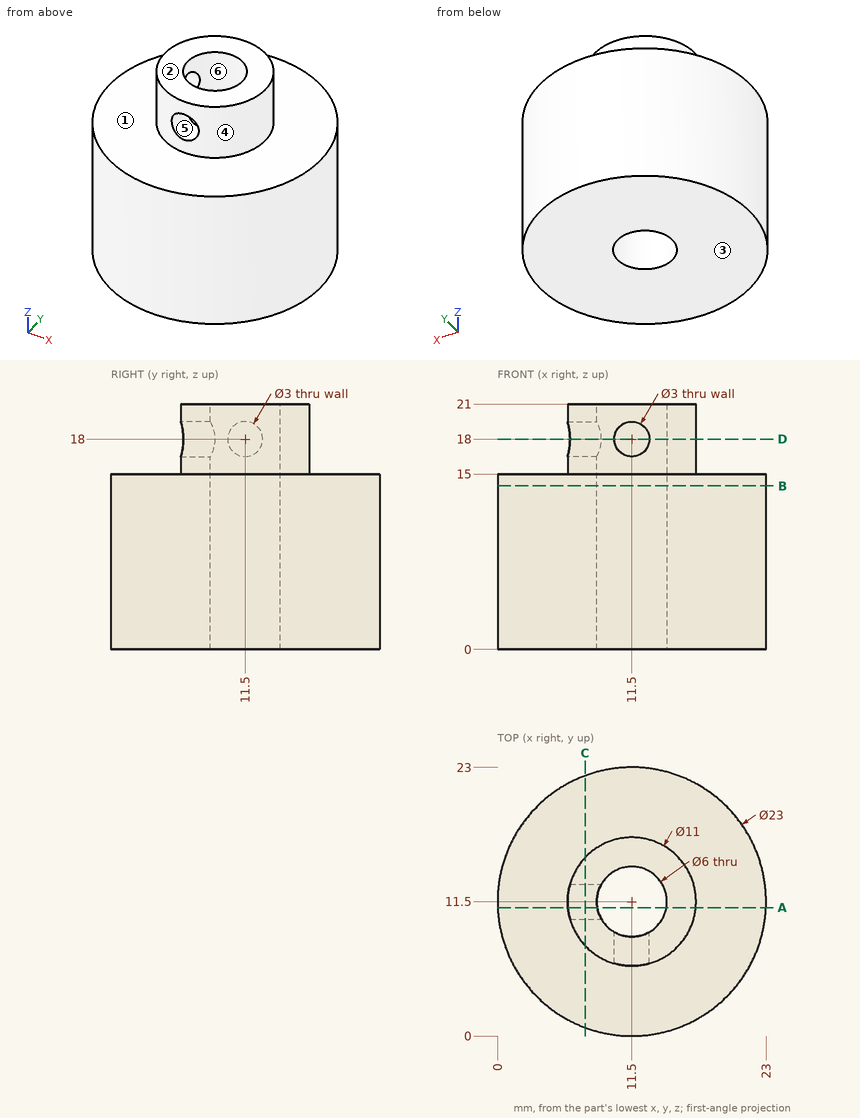
Check sheet for the drawn part. Datum: minimum x, y, z corner. Units: mm. A direction names the side the tool comes from. Round coordinates to 2 decimals unless told otherwise and drop trailing zeros. Order: outer loops, then holes, each group sorted by start corner. A loop starts at its lowest first (then second) coordinate and runs counter-clockwise, first axis right, second up.
(1) Cross-section at A-A, the plane y = 11. Enter the section's corners in (x, z).
(2) Access from +Z, -Z, +X, -X, +Y, -Y to the whole of each face (thin tool, end or side, straight path). Record for the marked faces 1 and 2.
(3) Cross-section at C-C, the plane x = 7.5. Enter the section's corners in (y, z).
(4) Cross-section at B-B, the plane z = 14. Enter the section's corners in (x, y), and give its area (3 significant figures).
(5) Go/stop test with flat-tipped pins: P1, Ø1, axis at x = 16, z = 17.5, coming from the +Y side; P2, Ø4, axis at y = 20.5, z = 10.5, coming from the -X side; P3, Ø10, axis at y = 17.5, z = 15.5, coming from the -X side. Record where each tip stops, or that it passes through.
(6) Draft check along X on the marked faces 3, 4, 5 and 6. Enter one of: pulls with the +X half, pulls with the -X half, needs draft (parallel to the pull), parting line crosses it, or undercut.
(7) Cross-section at D-D, the plane z = 18. Enter the section's corners in (x, y).
(8) Scan lines: probe 1 along Z at (x, y) = (11.5, 8.15); probe 2 along Z at (x, y) = (3, 10.75); probe 3 along Y at (x, z) = (13.25, 11.5). Record each from-to range of solid material in increasing order.
Check sheet entries:
1. outline: (0.01, 0) - (8.54, 0) - (8.54, 16.59) - (6.02, 16.59) - (6.02, 15) - (0.01, 15) - close; (6.02, 19.41) - (8.54, 19.41) - (8.54, 21) - (6.02, 21) - close; (14.46, 0) - (22.99, 0) - (22.99, 15) - (16.98, 15) - (16.98, 21) - (14.46, 21) - close
2. face 1: +Z
2. face 2: +Z, +X, -X, +Y, -Y
3. outline: (0.72, 0) - (22.28, 0) - (22.28, 15) - (15.27, 15) - (15.27, 21) - (7.73, 21) - (7.73, 15) - (0.72, 15) - close; hole circle Ø3 at (11.5, 18)
4. outline: circle Ø23 at (11.5, 11.5); hole circle Ø6 at (11.5, 11.5)
4. area: 387 mm2
5. P1: stops at y = 15.27
5. P2: stops at x = 2.38
5. P3: stops at x = 0.05
6. face 3: needs draft
6. face 4: parting line crosses it
6. face 5: undercut
6. face 6: undercut
7. outline: (6.21, 10) arc R5.5 ccw to (10, 6.21) - (10, 8.9) arc R3 cw to (8.9, 10) - close; (6.21, 13) - (8.9, 13) arc R3 cw (long way) to (13, 8.9) - (13, 6.21) arc R5.5 ccw (long way) to start
8. probe 1: z = 0 to 16.5, 19.5 to 21
8. probe 2: z = 0 to 15
8. probe 3: y = 0.13 to 9.06, 13.94 to 22.87
